Check sheet for the modelled part. Datum: model origin and axes. Units: mm. A direction names the side the tool comes from. Round coordinates to 2 decimals unless told otherwise and drop trailing zeros. Order: outer loops, then holes, each group sorted by start corner. A loop starts at its lowest first (then second) coordinate and runs counter-clockwise, first axis right, second up. Notation, with made-up numbers: (18, -20) -> (70, -20) arc R12 cw to (70, -12) -> close; hole circle Ø4 at (85, 3). An arc over 180 degrees is marked (long way). Answer in a Markdown table with one row per item.
from build123d import *

# Parameters (mm, degrees)
FILLET_1_R = 0.5


with BuildPart() as part:
    # Эскиз1 → Повернуть1 (revolve)
    with BuildSketch(Plane.XY):
        Polygon((-5.295963856, 0), (-7.091803279, 0), (-7.091803279, 0.5), (-6, 0.5), (-6, 2.5), (0, 2.5), (0, 1.340599242), (-5.295963856, 1.340599242), align=None)
    revolve(axis=Axis((0, 2.5, 0), (0, -1, 0)))

    # Скругление1
    fillet_1_edges = [part.edges().sort_by_distance(p)[0] for p in [
        (6, 2.5, 0),
    ]]
    fillet(fillet_1_edges, radius=FILLET_1_R)


solid = part.part
Item 1: Depth check by flat-ended pin: P1, Ø1, axis at x = -2.5, z = -2.5, coming from the -Y side; P2, Ø1, axis at y = 1.5, z = -1, coming from the -X side; P3, Ø1.5, axis at y = 1.5, z = -4.5, coming from the -X side. Enter the tip coordinate at first touch or a pass-through.
Result sheet:
| item | result |
|---|---|
| P1 | stops at y = 1.34 |
| P2 | stops at x = -5.98 |
| P3 | stops at x = -4.68 |
Item 2: Set-up check for faces 1 (the flat face through (-3, 0, 5)), 2 (the cylindrical face through (4.203, 0.661, 3.223)), 3 (the cylindrical face through (6, 1, 0)): record each of +Z, -Z, +X, -X, +Y, -Y from which the full face is reachable in a straight line by a thin tool's end or side.
Result sheet:
| item | result |
|---|---|
| face 1 | +Z, -Z, +X, -X, -Y |
| face 2 | -Y |
| face 3 | +Y |
Item 3: Cross-section at B-B (z = 0). Record the boundary of the cut face in (x, y), and give its area (3 significant figures).
Result sheet:
| item | result |
|---|---|
| outline | (-7.09, 0) -> (-5.3, 0) -> (-5.3, 1.34) -> (5.3, 1.34) -> (5.3, 0) -> (7.09, 0) -> (7.09, 0.5) -> (6, 0.5) -> (6, 2) arc R0.5 ccw to (5.5, 2.5) -> (-5.5, 2.5) arc R0.5 ccw to (-6, 2) -> (-6, 0.5) -> (-7.09, 0.5) -> close |
| area | 16.8 mm^2 |
Item 4: Scan lines: line 1 (X direction, y = 0.8, z = 0); line 2 (Y direction, x = 4, z = -1.25). Record each from-to range of solid material in increasing order. Write a range as [from, to].
Result sheet:
| item | result |
|---|---|
| line 1 | x = [-6, -5.3], [5.3, 6] |
| line 2 | y = [1.34, 2.5] |
Item 5: Cross-section at A-A (x = 0). Record the boundary of the cut face in (y, z), and give its area (3 significant figures).
Result sheet:
| item | result |
|---|---|
| outline | (0, -7.09) -> (0.5, -7.09) -> (0.5, -6) -> (2, -6) arc R0.5 ccw to (2.5, -5.5) -> (2.5, 5.5) arc R0.5 ccw to (2, 6) -> (0.5, 6) -> (0.5, 7.09) -> (0, 7.09) -> (0, 5.3) -> (1.34, 5.3) -> (1.34, -5.3) -> (0, -5.3) -> close |
| area | 16.8 mm^2 |
Item 6: Cross-section at C-C (y = 1.1). Record the boundary of the cut face in (x, z), and give its area (3 significant figures).
Result sheet:
| item | result |
|---|---|
| outline | circle Ø12 at (0, 0); hole circle Ø10.59 at (0, 0) |
| area | 25.0 mm^2 |
Item 7: Mould release check, pull along X, two halves, no side actions. Record for faces 4 (the flat face through (0, 1.341, 0)), 5 (the cylindrical face through (5.23, 0.25, -4.79)), 6 (the flat face through (0, 2.5, 0)): pulls with the +X half, pulls with the -X half, needs draft (parallel to the pull), parting line crosses it, or undercut.
Result sheet:
| item | result |
|---|---|
| face 4 | undercut |
| face 5 | parting line crosses it |
| face 6 | needs draft |
